Autodesk Fusion 360 part; units mm, degrees
sketch "스케치1" plane through (0, 0, 0) normal (0, 0, 1) x (1, 0, 0)
  line L0 (0, 0) -> (116, 0)
  line L1 (116, 0) -> (116, 30)
  line L2 (116, 30) -> (0, 30)
  line L3 (0, 30) -> (0, 0)
  dimension "d1" = 116
  dimension "d2" = 30
extrude "돌출1" add sketch "스케치1" along normal blind 5
fillet "필렛1" radius 15 4 edges at (0, 0, 2.5) (116, 0, 2.5) (116, 30, 2.5) (0, 30, 2.5)
sketch "스케치2" plane through (0, 0, 5) normal (0, 0, 1) x (-1, 0, 0)
  arc A0 (-15, -30) -> (-15, 0) centre (-15, -15) ccw
  line L0 (-15, 0) -> (-101, 0)
  arc A1 (-101, 0) -> (-101, -30) centre (-101, -15) ccw
  line L1 (-101, -30) -> (-15, -30)
  circle A2 centre (-58, -15) radius 10.95
  dimension "d7" = 15
  dimension "d8" = 58
  dimension "d9" = 21.9
extrude "돌출2" add sketch "스케치2" along normal blind 1.9
sketch "스케치3" plane through (0, 0, 5) normal (0, 0, 1) x (-1, 0, 0)
  circle A0 centre (-58, -15) radius 10.95
  circle A1 centre (-58, -15) radius 1.4
  circle A2 centre (-58, -15) radius 7.8085 construction
  circle A3 centre (-61.6659, -21.8945) radius 1
  circle A4 centre (-50.7199, -12.1763) radius 1
  circle A5 centre (-60.8237, -7.7199) radius 1
  line L0 (-61.6659, -21.8945) -> (-58, -15) construction
  line L1 (-58, -15) -> (-50.7199, -12.1763) construction
  line L2 (-58, -15) -> (-60.8237, -7.7199) construction
  line L3 (-58, -15) -> (-58, -25.95) construction
  dimension "d12" = 2.8
  dimension "d13" = 15.617
  dimension "d14" = 2
  dimension "d15" = 2
  dimension "d16" = 2
  dimension "d17" = 90
  dimension "d18" = 139.2
  dimension "d20" = 28
extrude "돌출3" cut sketch "스케치3" against normal blind 5 contours A1 | A3 | A4 | A5
equation "d8 = ( 116 / 2 ) * 1 mm"
Verification items for the finished model (mm, model axes). A direction names the side the tool comes from. Coordinates: 2 decimals unless noted, no trailing zeros. Order: outer loops, then holes, each group sorted by start corner. A loop starts at its lowest first (then second) coordinate and runs counter-clockwise, first axis right, second up. Notation, with made-up numbers: (-9, -13) -> (13, -13) arc R17 ccw to (13, 12) -> close; hole circle Ø7 at (35.5, -0.75). An arc over 180 degrees is marked (long way). Put each result on its own line as item: value. Start each with the question number.
1. Cross-section at B-B, the plane z = 1.75. Count the separate pieces of the cut face and the enclosed holes in it, then the cut area to 3 significant figures.
2. Access from +Z, -Z, +X, -X, +Y, -Y to the whole of each face (thin tool, end or side, straight path). Record for faces 1 (the flat face through (59, 30, 3)), 2 (the cylindrical face through (66.69, 8.34, 5.94)).
3. Cross-section at A-A, the plane x = 58. Record the boundary of the cut face in (y, z).
4. Material ranges on L1, parallel to X at y = 15, z = 6.05; L2, parallel to Y at x = 58, z = 3.75; L3, parallel to X at y = 8, z = 1.25, recorded low to high. Write a range as [from, to].
5. Go/stop test with flat-tipped pins: pin 1 Ø3.5 at (x, y) = (58, 15) entering from -Z; pin 2 Ø11 at (x, y) = (57.5, 12.5) entering from +Z; pin 3 Ø4 at (y, z) = (26.5, 2.5) entering from +X. Record where each tip stops, or that it passes through.
6. Mould release check, pull along Y, two halves, no side actions. Record for faces 3 (the flat face through (46, 15, 6.9)), 4 (the cylindrical face through (111.49, 4.277, 2.535)), 5 (the cylindrical face through (61.823, 7.676, 2.535)): released by +Y, released by -Y, zero draft, split by the parting line, or undercut.
Computed:
1. separate pieces: 1
1. enclosed holes: 4
1. area: 3,270 mm2
2. face 1: +Z, -Z, +X, -X, +Y
2. face 2: +Z
3. outline: (0, 0) -> (13.6, 0) -> (13.6, 5) -> (4.05, 5) -> (4.05, 6.9) -> (0, 6.9) -> close; (16.4, 0) -> (30, 0) -> (30, 6.9) -> (25.95, 6.9) -> (25.95, 5) -> (16.4, 5) -> close
4. L1: [0, 47.05], [68.95, 116]
4. L2: [0, 13.6], [16.4, 30]
4. L3: [1.73, 59.86], [61.78, 114.27]
5. pin 1: z = 0
5. pin 2: z = 5
5. pin 3: x = 112.61
6. face 3: zero draft
6. face 4: released by -Y
6. face 5: undercut
